Study the drawing (mm; zero at the part's minimum x, y, z) and answer. A direction names the side the tool comes from. Coordinates: 2 decimals unless noted, no trailing zeros. Write each loop counter-clockwise with the first axis right and the second up, starting at its lowest first coordinate (ties: lowest second). Pieces come first, ordered by that corner, then holes. Notation, with made-up numbers: (32.25, 62.25) -> (62.25, 62.25) arc R14 cw to (62.25, 71.25) -> close; hole circle Ø5 at (30, 33). An arc over 180 degrees is marked (long way). Write each question's results on one line, items separated by ' | '. Start each with the question number.
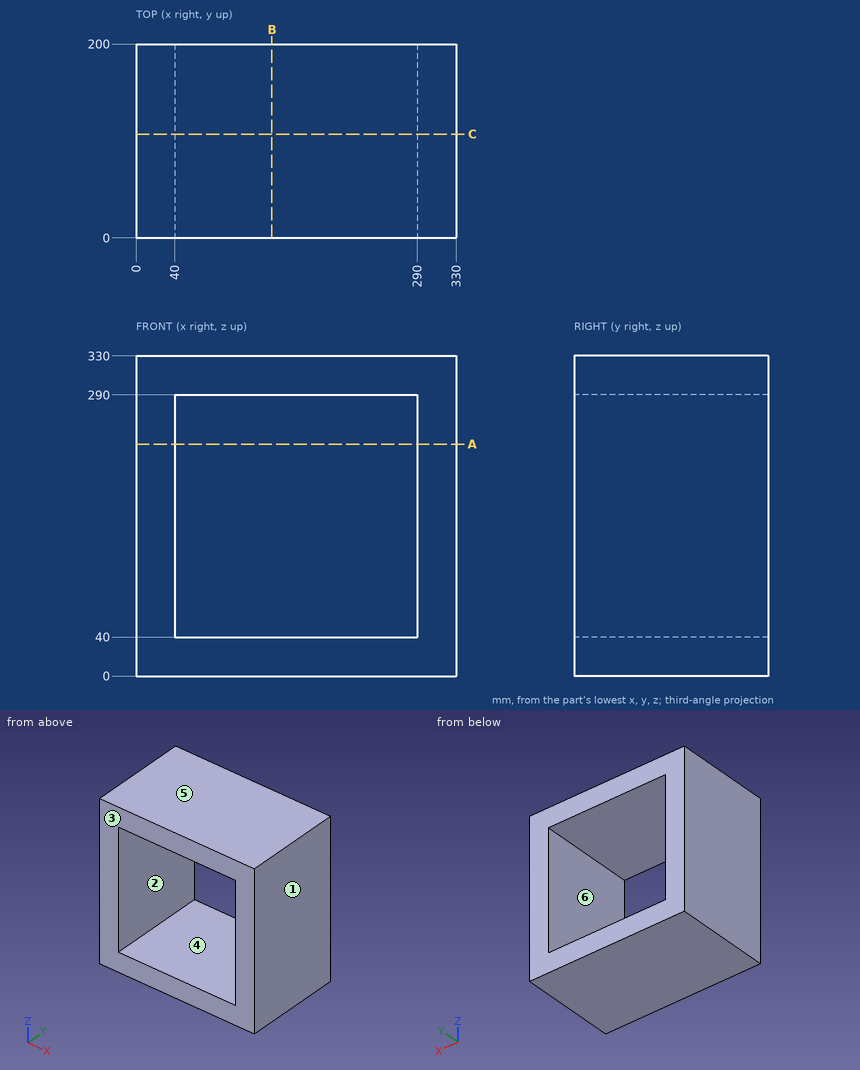
1. For the marked faces 1 and 2, determine the directions among +Z, -Z, +X, -X, +Y, -Y from which every point of the face is accessible in a straight line to the end or side of a thin tool.
2. Find section A-A on z = 239. Give the vertices of the cut face in (x, y), and give its area (3 significant figures).
3. Find the intervals of material crossed by L1, parallel to X at y = 186.5, z = 250.5, in increasing order.
4. Determine the mould class of the marked faces 3, 4, 5 and 6 for opening direction Z: pulls with the +Z half, pulls with the -Z half, needs draft (parallel to the pull), parting line crosses it, or undercut.
5. Find section B-B on x = 140. Give the vertices of the cut face in (y, z).
6. Find section C-C on y = 107. Give the vertices of the cut face in (x, z).
Ans:
1) face 1: +Z, -Z, +X, +Y, -Y | face 2: +Y, -Y
2) outline: (0, 0) -> (40, 0) -> (40, 200) -> (0, 200) -> close; (290, 0) -> (330, 0) -> (330, 200) -> (290, 200) -> close | area: 16,000 mm²
3) L1: x = 0 to 40, 290 to 330
4) face 3: needs draft | face 4: undercut | face 5: pulls with the +Z half | face 6: undercut
5) outline: (0, 0) -> (200, 0) -> (200, 40) -> (0, 40) -> close; (0, 290) -> (200, 290) -> (200, 330) -> (0, 330) -> close
6) outline: (0, 0) -> (330, 0) -> (330, 330) -> (0, 330) -> close; hole (40, 40) -> (290, 40) -> (290, 290) -> (40, 290) -> close
